from build123d import *

# Parameters (mm, degrees)
GUIDED_START                               = 38.4
SKETCH1_W                                  = 12
SKETCH1_H                                  = 40
GUIDED_BRIDGE_WITH_ROD_COUPLING_SEAT_DEPTH = 23.2
LOWER_START                                = 38.4
SKETCH2_W                                  = 19
SKETCH2_H                                  = 49
LOWER_RACK_LAP_DEPTH                       = 4
UPPER_START                                = 57.6
SKETCH3_W                                  = 19
SKETCH3_H                                  = 49
UPPER_RACK_LAP_DEPTH                       = 4
M4_START                                   = 38.4
SKETCH4_R                                  = 2.15
M4_JOINT_BOLT_CLEARANCE_DEPTH              = 23.2
RADIAL_START                               = 65
SKETCH5_R                                  = 6.15
RADIAL_FLOATING_STUD_CLEARANCE_DEPTH       = 12


with BuildPart() as part:
    # Sketch1 → Guided bridge with rod coupling seat (new body)
    with BuildSketch(Plane.XY.offset(GUIDED_START)):
        with Locations((71, 64)):
            Rectangle(SKETCH1_W, SKETCH1_H)
    extrude(amount=GUIDED_BRIDGE_WITH_ROD_COUPLING_SEAT_DEPTH)

    # Sketch2 → Lower rack lap (add)
    with BuildSketch(Plane.XY.offset(LOWER_START)):
        with Locations((67.5, 59.5)):
            Rectangle(SKETCH2_W, SKETCH2_H)
    extrude(amount=LOWER_RACK_LAP_DEPTH)

    # Sketch3 → Upper rack lap (add)
    with BuildSketch(Plane.XY.offset(UPPER_START)):
        with Locations((67.5, 59.5)):
            Rectangle(SKETCH3_W, SKETCH3_H)
    extrude(amount=UPPER_RACK_LAP_DEPTH)

    # Sketch4 → M4 joint bolt clearance (cut)
    with BuildSketch(Plane.XY.offset(M4_START)):
        with Locations((60.5, 38.8)):
            Circle(SKETCH4_R)
        with Locations((69.5, 38.8)):
            Circle(SKETCH4_R)
    extrude(amount=M4_JOINT_BOLT_CLEARANCE_DEPTH, mode=Mode.SUBTRACT)

    # Sketch5 → Radial floating stud clearance (cut)
    with BuildSketch(Plane(origin=(0, 0, 0), x_dir=(0, 0, -1), z_dir=(1, 0, 0)).offset(RADIAL_START)):
        with Locations((-50, 69)):
            Circle(SKETCH5_R)
    extrude(amount=RADIAL_FLOATING_STUD_CLEARANCE_DEPTH, mode=Mode.SUBTRACT)


solid = part.part
Input: part model. Units: mm. Frame: model coordinates. A direction names the side the tool comes from. Give positions to 0.01 mm unless a question says otherwise; leave off trailing zeros. Loops run counter-clockwise (first coordinate to the right, second up) from the corner with the lowest first, then second, coordinate; pieces in that order, holes last. Notation, with made-up numbers: (-37.75, 78.5) -> (-13.75, 78.5) arc R21 ccw to (-13.75, 103.5) -> close; hole circle Ø5 at (-0.5, -9). An arc over 180 degrees is marked (long way). Answer as a JSON object with one key per item and string values. Group by question number.
Item 1: Pull-direction query (X, two-part tool) for faces 4 (the cylindrical face through (58.794, 37.492, 59.572)), 5 (the flat face through (65, 59, 50)), 6 (the flat face through (67, 35, 60)); classes: released by +X, released by -X, zero draft, split by the parting line, or undercut.
Item 2: Pin query (flat end, axial travel): P1, Ø3.5, axis at x = 60.5, y = 38.8, coming from the -Z side; P2, Ø8, axis at x = 64, z = 49, coming from the -Y side; P3, Ø8, axis at y = 45.5, z = 52.5, coming from the -X side. Return the tip coordinate at first contact, or that it passes through.
Item 3: Cut plane A-A, the plane x = 60.5. Return the cut outline in (y, z), and give its area (3 significant figures).
Item 4: Cut plane B-B, the plane y = 69. Return the cut outline in (x, z).
Item 5: Line query: probe 1 along X at (y, z) = (38.8, 40.15); probe 2 along Y at (x, z) = (69.5, 59.75); probe 3 along Z at (x, y) = (62, 67). Output: solid intervals per line, ascending.
Item 6: Cut plane C-C, the plane x = 69.5. Return the cut outline in (y, z), and give its area (3 significant figures).
Item 7: Cut plane D-D, the plane y = 38.8. Return the cut outline in (x, z), and give its area (3 significant figures).
Item 8: Reachability of faces 1 (the flat face through (71, 44, 50)), 2 (the flat face through (63, 54, 57.6)), 3 (the flat face through (67, 35, 40)) from +Z, -Z, +X, -X, +Y, -Y: full face, straight path, thin tool, end or side. Return the list, or none.
Checks:
{
 "1": {"face 4": "undercut", "face 5": "released by -X", "face 6": "zero draft"},
 "2": {"P1": "passes through", "P2": "stops at y = 44", "P3": "stops at x = 65"},
 "3": {"outline": "(35, 38.4) -> (36.65, 38.4) -> (36.65, 42.4) -> (35, 42.4) -> close; (35, 57.6) -> (36.65, 57.6) -> (36.65, 61.6) -> (35, 61.6) -> close; (40.95, 38.4) -> (84, 38.4) -> (84, 42.4) -> (40.95, 42.4) -> close; (40.95, 57.6) -> (84, 57.6) -> (84, 61.6) -> (40.95, 61.6) -> close", "area": "358 mm²"},
 "4": {"outline": "(58, 38.4) -> (77, 38.4) -> (77, 43.85) -> (65, 43.85) -> (65, 42.4) -> (58, 42.4) -> close; (58, 57.6) -> (65, 57.6) -> (65, 56.15) -> (77, 56.15) -> (77, 61.6) -> (58, 61.6) -> close"},
 "5": {"probe 1": "x = 58 to 58.35, 62.65 to 67.35, 71.65 to 77", "probe 2": "y = 35 to 36.65, 40.95 to 84", "probe 3": "z = 38.4 to 42.4, 57.6 to 61.6"},
 "6": {"outline": "(35, 38.4) -> (36.65, 38.4) -> (36.65, 42.4) -> (35, 42.4) -> close; (35, 57.6) -> (36.65, 57.6) -> (36.65, 61.6) -> (35, 61.6) -> close; (40.95, 38.4) -> (84, 38.4) -> (84, 61.6) -> (40.95, 61.6) -> (40.95, 57.6) -> (44, 57.6) -> (44, 42.4) -> (40.95, 42.4) -> close; hole circle Ø12.3 at (69, 50)", "area": "847 mm²"},
 "7": {"outline": "(58, 38.4) -> (58.35, 38.4) -> (58.35, 42.4) -> (58, 42.4) -> close; (58, 57.6) -> (58.35, 57.6) -> (58.35, 61.6) -> (58, 61.6) -> close; (62.65, 38.4) -> (67.35, 38.4) -> (67.35, 42.4) -> (62.65, 42.4) -> close; (62.65, 57.6) -> (67.35, 57.6) -> (67.35, 61.6) -> (62.65, 61.6) -> close; (71.65, 38.4) -> (77, 38.4) -> (77, 42.4) -> (71.65, 42.4) -> close; (71.65, 57.6) -> (77, 57.6) -> (77, 61.6) -> (71.65, 61.6) -> close", "area": "83.2 mm²"},
 "8": {"face 1": "+X, -X, -Y", "face 2": "-X, -Y", "face 3": "+Z, -Z, +X, -X, -Y"}
}
